Autodesk Inventor part; units mm, degrees
ref_plane "YZ Plane" through (0, 0, 0) normal (1, 0, 0) x (0, 1, 0)
ref_plane "XZ Plane" through (0, 0, 0) normal (0, 1, 0) x (-1, 0, 0)
ref_plane "XY Plane" through (0, 0, 0) normal (0, 0, 1) x (1, 0, 0)
sketch "Sketch44" plane through (0, 0, 0) normal (0, 1, 0) x (-1, 0, 0)
  line L0 (-39.5, 120) -> (39.5, 120)
  line L1 (39.5, 120) -> (39.5, -120)
  line L2 (39.5, -120) -> (-39.5, -120)
  line L3 (-39.5, -120) -> (-39.5, 120)
  line L4 (-39.5, 120) -> (39.5, -120) construction
  line L5 (39.5, 120) -> (-39.5, -120) construction
  point P0 (0, 0)
  dimension "d138" = 79
  dimension "d139" = 240
extrude "Extrusion33" add sketch "Sketch44" along normal blind 3
sketch "Sketch45" plane through (0, 3, 0) normal (0, 1, 0) x (1, 0, 0)
  line L0 (35, -20) -> (-3, -20)
  line L1 (-3, -20) -> (-3, 20)
  line L2 (-3, 20) -> (35, 20)
  line L3 (35, 20) -> (35, -20)
  point P0 (0, 0)
  dimension "d142" = 38
  dimension "d143" = 40
extrude "Extrusion34" add sketch "Sketch45" along normal blind 30
sketch "Sketch47" plane through (0, 0, 0) normal (0, -1, 0) x (1, 0, 0)
  circle A0 centre (16, 0) radius 18
  point P0 (0, 0)
  dimension "d146" = 36
extrude "Extrusion35" cut sketch "Sketch47" against normal blind 30 draft -15
sketch "Sketch58" plane through (35, 3, -20) normal (0, 0, -1) x (-1, 0, 0)
  line L0 (7, 20) -> (27, 20)
  line L1 (27, 20) -> (27, 5)
  line L2 (27, 5) -> (7, 5)
  line L3 (7, 5) -> (7, 20)
  point P0 (35, -3)
  dimension "d156" = 20
  dimension "d157" = 15
extrude "Extrusion38" cut sketch "Sketch58" against normal blind 15
sketch "Sketch59" plane through (-3, 3, -20) normal (-1, 0, 0) x (0, 0, 1)
  line L0 (4.8, 25) -> (8, 25)
  line L1 (8, 25) -> (8, 5)
  line L2 (8, 5) -> (4.8, 5)
  line L3 (4.8, 5) -> (4.8, 25)
  point P0 (20, -3)
  dimension "d160" = 3.2
  dimension "d161" = 20
extrude "Extrusion39" cut sketch "Sketch59" against normal blind 35
sketch "Sketch60" plane through (0, 3, 0) normal (0, 1, 0) x (1, 0, 0)
  line L0 (-33.965, 38.3247) -> (-28.965, 38.3247)
  line L1 (-28.965, 38.3247) -> (-28.965, 58.3247)
  line L2 (-28.965, 58.3247) -> (-33.965, 58.3247)
  line L3 (-33.965, 58.3247) -> (-33.965, 38.3247)
  point P0 (0, 0)
  dimension "d164" = 5
  dimension "d165" = 20
extrude "Extrusion40" add sketch "Sketch60" along normal blind 20
sketch "Sketch61" plane through (0, 23, 0) normal (0, 1, 0) x (1, 0, 0)
  line L0 (-28.965, 38.3247) -> (-28.965, 58.3247)
  line L1 (-28.965, 38.3247) -> (-48.965, 38.3247)
  line L2 (-48.965, 38.3247) -> (-48.965, 58.3247)
  line L3 (-48.965, 58.3247) -> (-28.965, 58.3247)
  line L4 (-28.965, 58.3247) -> (-28.965, 38.3247)
  point P0 (0, 0)
  dimension "d168" = 20
  dimension "d169" = 20
extrude "Extrusion41" add sketch "Sketch61" against normal blind 5
sketch "Sketch64" plane through (0, 33, 0) normal (0, 1, 0) x (1, 0, 0)
  circle A0 centre (20, 0) radius 1
  point P0 (0, 0)
  dimension "d173" = 2
extrude "Extrusion42" cut sketch "Sketch64" against normal through all
sketch "Sketch65" plane through (-3, 3, -20) normal (-1, 0, 0) x (0, 0, 1)
  circle A0 centre (20, 15) radius 3
  point P0 (20, -3)
  dimension "d176" = 6
extrude "Extrusion43" cut sketch "Sketch65" against normal blind 10
sketch "Sketch68" plane through (0, 3, 0) normal (0, 1, 0) x (1, 0, 0)
  circle A0 centre (-31.5, -112) radius 3.5
  circle A1 centre (31.5, -112) radius 3.5
  circle A2 centre (-31.5, 112) radius 3.5
  circle A3 centre (31.5, 112) radius 3.5
  point P0 (0, 0)
  dimension "d192" = 7
  dimension "d193" = 7
  dimension "d194" = 7
  dimension "d195" = 7
extrude "Extrusion46" cut sketch "Sketch68" against normal through all
sketch "Sketch69" plane through (0, 3, 0) normal (0, 1, 0) x (1, 0, 0)
  circle A0 centre (23.5, -27) radius 3.5
  circle A1 centre (23.5, 27) radius 3.5
  point P0 (0, 0)
  dimension "d198" = 7
  dimension "d199" = 7
extrude "Extrusion47" cut sketch "Sketch69" against normal through all
sketch "Sketch70" plane through (0, 0, 0) normal (0, -1, 0) x (1, 0, 0)
  line L0 (-3, -12) -> (32, -12)
  line L1 (2.479, -12) -> (29.6644, -12)
  line L2 (29.6644, -12) -> (29.6644, -18.105)
  line L3 (29.6644, -18.105) -> (2.479, -18.105)
  line L4 (2.479, -18.105) -> (2.479, -12)
  point P0 (0, 0)
extrude "Extrusion48" add sketch "Sketch70" against normal blind 8
equation "\"d193\" = d192"
equation "\"d194\" = d192"
equation "\"d195\" = d192"
equation "\"d198\" = d192"
equation "\"d199\" = d192"
properties part number "liquid port_v07"
Work out the finished part from the listing and answer in its coordinate system (mm). A direction names the side the tool comes from. Give positions to 0.01 mm unless a question says otherwise; leave off trailing zeros. Loops run counter-clockwise (first coordinate to the right, second up) from the corner with the lowest first, then second, coordinate; pieces in that order, holes last. Notation, with made-up numbers: (26, -31) - (81, -31) arc R7 cw to (81, -18) - close; hole circle Ø10 at (52, -26.75). An arc over 180 degrees is marked (long way). Use CSV: the item, a comma, the result in double quotes. Start each with the question number.
(1) Find section A-A, the plane z = -112. Determine the outline of the cut face in (x, y).
(2) Find the intervals of material crossed by L1, parallel to X at y = 1, z = -112; L2, parallel to Z at x = 31, y = 18; L3, parallel to X at y = 1, z = 27, in increasing order.
(3) A tool of negligible diameter and unlimited length cuts with its end or side. For faces 1 (the face through (16, 18, 20)), 2 (the face through (16, 30, 0)), 3 (the face through (16, 24, -20)), 4 (the face through (28, 15, -18)), from which of +Z, -Z, +X, -X, +Y, -Y can it reach the whole face along a straight path? Write none if from no direction.
(4) Find section B-B, the plane x = -31.5. Determine the outline of the cut face in (y, z), plus the area to 3 significant figures.
(5) Each of these flat-tipped pins is pushed along its axis until it touches: pin 1 (10 mm diameter, centred on x = 6.5, z = -71, fed in from +Y); pin 2 (4 mm diameter, centred on y = 12, z = -17, fed in from -X); pin 3 (16 mm diameter, centred on x = -40.5, y = 17, fed in from +Z); pin 4 (12 mm diameter, centred on y = 6, z = -23.5, fed in from +X). Where does it stop, or does it pass through?
(6) Find section C-C, the plane z = -41. Determine the outline of the cut face in (x, y) (3 decimals), plus the area to 3 significant figures.
(7) Find section D-D, the plane z = 27. Determine the outline of the cut face in (x, y), plus the area to 3 significant figures.
(8) Determine the mould class of faces 5 (the face through (16, 33, 0)), 6 (the face through (6, 20, -15.2)), 7 (the face through (-48.965, 21, -48)) for opening direction Y: released by +Y, released by -Y, zero draft, split by the parting line, or undercut.
Results found:
1,outline,"(-39.5, 0) - (-35, 0) - (-35, 3) - (-39.5, 3) - close; (-28, 0) - (28, 0) - (28, 3) - (-28, 3) - close; (35, 0) - (39.5, 0) - (39.5, 3) - (35, 3) - close"
2,L1,"-39.5 to -35, -28 to 28, 35 to 39.5"
2,L2,"-20 to -15.2, -12 to 20"
2,L3,"-39.5 to 20, 27 to 39.5"
3,face 1,"+Z, +X, -X, +Y"
3,face 2,"-Y"
3,face 3,"-Z, +X, -X, +Y"
3,face 4,"-Z"
4,outline,"(0, -120) - (3, -120) - (3, -115.5) - (0, -115.5) - close; (0, -108.5) - (3, -108.5) - (3, -58.32) - (23, -58.32) - (23, -38.32) - (3, -38.32) - (3, 108.5) - (0, 108.5) - close; (0, 115.5) - (3, 115.5) - (3, 120) - (0, 120) - close"
4,area,"1,080 mm^2"
5,pin 1,"y = 3"
5,pin 2,"x = -3"
5,pin 3,"z = -38.32"
5,pin 4,"x = 39.5"
6,outline,"(-48.965, 18) - (-33.965, 18) - (-33.965, 3) - (-39.5, 3) - (-39.5, 0) - (39.5, 0) - (39.5, 3) - (-28.965, 3) - (-28.965, 23) - (-48.965, 23) - close"
6,area,"412 mm^2"
7,outline,"(-39.5, 0) - (20, 0) - (20, 3) - (-39.5, 3) - close; (27, 0) - (39.5, 0) - (39.5, 3) - (27, 3) - close"
7,area,"216 mm^2"
8,face 5,"released by +Y"
8,face 6,"undercut"
8,face 7,"zero draft"
